```python
from build123d import *

# Parameters (mm, degrees)
SKETCH1_W           = 45
SKETCH1_H           = 80
SKETCH1_W_2         = 25.5
SKETCH1_H_2         = 40.7
BOSS_EXTRUDE1_DEPTH = 3.1
SKETCH8_W           = 45
SKETCH8_H           = 15.85
CUT_EXTRUDE4_DEPTH  = 4.1


with BuildPart() as part:
    # Sketch1 → Boss-Extrude1 (new body)
    with BuildSketch(Plane.XY):
        Rectangle(SKETCH1_W, SKETCH1_H)
        with Locations((0, -10.35)):
            Rectangle(SKETCH1_W_2, SKETCH1_H_2, mode=Mode.SUBTRACT)
        with BuildLine():
            Line((-10.115047428, 16.65), (9.493300094, 16.65))
            ThreePointArc((9.493300094, 16.65), (12.550371011, 14.101497401), (9.398611565, 11.671073469))
            Line((9.398611565, 11.671073469), (-10.115047428, 11.65))
            ThreePointArc((-10.115047428, 11.65), (-12.502645782, 14.15), (-10.115047428, 16.65))
        make_face(mode=Mode.SUBTRACT)
        with BuildLine():
            Line((-10.115047428, -32.35), (9.398611565, -32.371073469))
            ThreePointArc((9.398611565, -32.371073469), (12.550371011, -34.801497401), (9.493300094, -37.35))
            Line((9.493300094, -37.35), (-10.115047428, -37.35))
            ThreePointArc((-10.115047428, -37.35), (-12.502645782, -34.85), (-10.115047428, -32.35))
        make_face(mode=Mode.SUBTRACT)
    extrude(amount=BOSS_EXTRUDE1_DEPTH)

    # Sketch8 → Cut-Extrude4 (cut, through all)
    with BuildSketch(Plane.XY.offset(3.1)):
        with Locations((0, 32.075)):
            Rectangle(SKETCH8_W, SKETCH8_H)
    extrude(amount=-CUT_EXTRUDE4_DEPTH, mode=Mode.SUBTRACT)


solid = part.part
```
Geometry check sheet. Reference: the model listing, model coordinates, mm. A direction names the side the tool comes from. Give positions to 0.01 mm unless a question says otherwise; leave off trailing zeros. Order: outer loops, then holes, each group sorted by start corner. A loop starts at its lowest first (then second) coordinate and runs counter-clockwise, first axis right, second up. Notation, with made-up numbers: (60.25, -9.5) - (98.25, -9.5) arc R7 cw to (98.25, -1.5) - close; hole circle Ø8 at (68, 50.5). An arc over 180 degrees is marked (long way). Answer in a Markdown table with one row per item. Add a question column.
Q1. Cross-section at A-A, the plane y = 6. Enter the section's corners in (x, z), then the cut area to 4 significant figures.
Q2. Mould release check, pull along X, two halves, no side actions. Record for faces 1 (the cylindrical face through (-12.502, 14.097, 1.528)), 2 (the flat face through (22.5, -8, 2)), 3 (the flat face through (0, -40, 2)): pulls with the +X half, pulls with the -X half, needs draft (parallel to the pull), parting line crosses it, or undercut.
Q3. Material ranges on probe 1 along Y at (x, z) = (10, 0.75); probe 2 along Y at (x, z) = (8.5, 2.55); probe 3 along X at (y, z) = (-34.85, 1.35), recorded low to high. Write a range as from..to.
Q4. Cross-section at D-D, the plane y = 14.15. Enter the section's corners in (x, z), then the cut area to 3 significant figures.
Q5. Cross-section at C-C, the plane x = 2. Enter the section's corners in (y, z).
Q6. Tool access check on faces 4 (the flat face through (-15, -7, 0)), 5 (the flat face through (12.75, -11, 2)). Record the directions out of +Z, -Z, +X, -X, +Y, -Y that give a thin tool (end or side, any length) a straight path to the whole face; none if there is none.
Q7. Cross-section at B-B, the plane z = 0.75. Enter the section's corners in (x, y).
Q8. Gauge pin test, flat end, axial feed: pin 1 (6 mm diameter, centred on x = 13, y = 11.5, fed in from -Z). Record the tip position at first contact, or that the pin passes through.
Check values:
| question | item | result |
|---|---|---|
| 1 | outline | (-22.5, 0) - (-12.75, 0) - (-12.75, 3.1) - (-22.5, 3.1) - close; (12.75, 0) - (22.5, 0) - (22.5, 3.1) - (12.75, 3.1) - close |
| 1 | area | 60.45 mm^2 |
| 2 | face 1 | undercut |
| 2 | face 2 | pulls with the +X half |
| 2 | face 3 | needs draft |
| 3 | probe 1 | y = -40..-37.4, -32.3..-30.7, 10..11.6, 16.7..24.15 |
| 3 | probe 2 | y = -40..-37.35, -32.37..-30.7, 10..11.67, 16.65..24.15 |
| 3 | probe 3 | x = -22.5..-12.5, 12.55..22.5 |
| 4 | outline | (-22.5, 0) - (-12.5, 0) - (-12.5, 3.1) - (-22.5, 3.1) - close; (12.55, 0) - (22.5, 0) - (22.5, 3.1) - (12.55, 3.1) - close |
| 4 | area | 61.8 mm^2 |
| 5 | outline | (-40, 0) - (-37.35, 0) - (-37.35, 3.1) - (-40, 3.1) - close; (-32.36, 0) - (-30.7, 0) - (-30.7, 3.1) - (-32.36, 3.1) - close; (10, 0) - (11.66, 0) - (11.66, 3.1) - (10, 3.1) - close; (16.65, 0) - (24.15, 0) - (24.15, 3.1) - (16.65, 3.1) - close |
| 6 | face 4 | -Z, +X, -X, +Y, -Y |
| 6 | face 5 | +Z, -Z |
| 7 | outline | (-22.5, -40) - (22.5, -40) - (22.5, 24.15) - (-22.5, 24.15) - close; hole (-12.75, -30.7) - (12.75, -30.7) - (12.75, 10) - (-12.75, 10) - close; hole (-10.12, -37.35) - (9.49, -37.35) arc R2.55 ccw (long way) to (9.4, -32.37) - (-10.12, -32.35) arc R2.5 ccw to start; hole (-10.12, 11.65) - (9.4, 11.67) arc R2.55 ccw (long way) to (9.49, 16.65) - (-10.12, 16.65) arc R2.5 ccw to start |
| 8 | pin 1 | stops at z = 0 |
